Input: part model. Units: mm. Frame: model coordinates. Give positions to 0.01 mm unless a question says otherwise; leave off trailing zeros. Loops run counter-clockwise (first coordinate to the right, second up) from the corner with the lowest first, then second, coordinate; pieces in that order, holes last. Notation, with made-up numbers: (83.25, 22) - (139.25, 22) arc R7 cw to (139.25, 35) - close; hole circle Ø1 at (75, 40). An arc over 180 degrees is marked (long way). Answer as a JSON object with one key per item and string values. Group by question number.
(1) Section query A-A (x = 0). Return loops of the section in (y, z).
(2) Pin query (flat end, axial travel): P1, Ø4.5, axis at x = 0, z = 11.5, coming from the -Y side. Return the tip coordinate at first contact, or that it passes through.
(3) Material intervals for L1, parallel to Y at x = 0, z = -22; L2, parallel to X at y = 8.5, z = -73.5, sorted ascending.
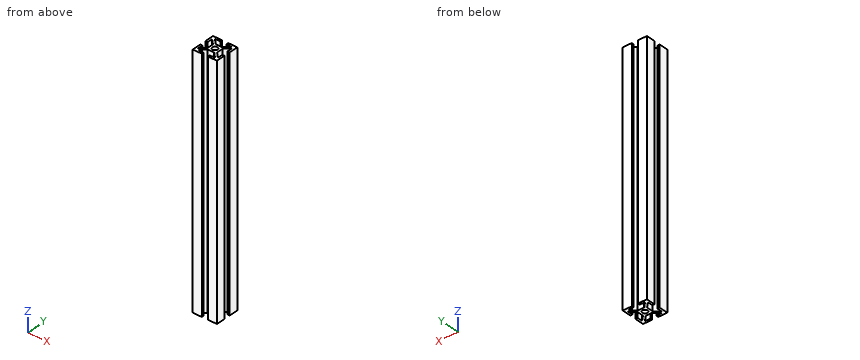
```python
from build123d import *

# Parameters (mm, degrees)
SKETCH2_R           = 2.15
BOSS_EXTRUDE1_DEPTH = 100


with BuildPart() as part:
    # Sketch2 → Boss-Extrude1 (new body, symmetric)
    with BuildSketch(Plane.XY):
        Polygon((-2.5, 10), (-2.5, 8.2), (-6.927207794, 8.2), (-2.677207794, 3.95), (2.677207794, 3.95), (6.927207794, 8.2), (2.5, 8.2), (2.5, 10), (10, 10), (10, 2.5), (8.2, 2.5), (8.2, 6.927207794), (3.95, 2.677207794), (3.95, -2.677207794), (8.2, -6.927207794), (8.2, -2.5), (10, -2.5), (10, -10), (2.5, -10), (2.5, -8.2), (6.927207794, -8.2), (2.677207794, -3.95), (-2.677207794, -3.95), (-6.927207794, -8.2), (-2.5, -8.2), (-2.5, -10), (-10, -10), (-10, -2.5), (-8.2, -2.5), (-8.2, -6.927207794), (-3.95, -2.677207794), (-3.95, 2.677207794), (-8.2, 6.927207794), (-8.2, 2.5), (-10, 2.5), (-10, 10), align=None)
        Circle(SKETCH2_R, mode=Mode.SUBTRACT)
    extrude(amount=BOSS_EXTRUDE1_DEPTH, both=True)


solid = part.part
```
Recorded:
{
 "1": {"outline": "(-3.95, -100) - (-2.15, -100) - (-2.15, 100) - (-3.95, 100) - close; (2.15, -100) - (3.95, -100) - (3.95, 100) - (2.15, 100) - close"},
 "2": {"P1": "stops at y = -3.95"},
 "3": {"L1": "y = -3.95 to -2.15, 2.15 to 3.95", "L2": "x = -10 to -2.5, 2.5 to 10"}
}
